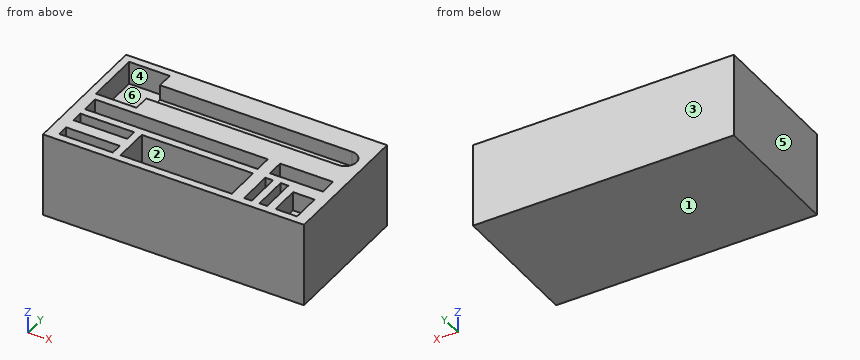
```python
from build123d import *

# Parameters (mm, degrees)
F0_W      = 340
F0_H      = 180
F1_DEPTH  = 110
F2_W      = 53
F2_H      = 72
F4_DEPTH  = 30
F5_DEPTH  = 20
F7_W      = 225
F7_H      = 22
F12_DEPTH = 100
F6_W      = 70
F6_H      = 15
F13_DEPTH = 80
F8_W      = 145
F8_H      = 46
F14_DEPTH = 100
F9_W      = 69
F9_H      = 22
F15_DEPTH = 100
F10_W     = 10
F10_H     = 46
F16_DEPTH = 15
F11_W     = 28
F11_H     = 38
F17_DEPTH = 25


with BuildPart() as f1:
    # F0 (on Top) → F1 (new body)
    with BuildSketch(Plane.XY):
        Rectangle(F0_W, F0_H)
    extrude(amount=-F1_DEPTH)

    # F2 (on face) → F4 (cut)
    with BuildSketch(Plane.XY):
        with Locations((-133.5, 44)):
            Rectangle(F2_W, F2_H)
    extrude(amount=-F4_DEPTH, mode=Mode.SUBTRACT)

    # F3 (on face) → F5 (cut)
    with BuildSketch(Plane.XY):
        with BuildLine():
            Line((143, 59), (-107, 59))
            Line((-107, 59), (-107, 29))
            Line((-107, 29), (143, 29))
            ThreePointArc((143, 29), (158, 44), (143, 59))
        make_face()
    extrude(amount=-F5_DEPTH, mode=Mode.SUBTRACT)

    # F7 (on face) → F12 (cut)
    with BuildSketch(Plane.XY):
        with Locations((-42.5, -13)):
            Rectangle(F7_W, F7_H)
    extrude(amount=-F12_DEPTH, mode=Mode.SUBTRACT)

    # F6 (on face) → F13 (cut)
    with BuildSketch(Plane.XY):
        with Locations((-120, -72.5)):
            Rectangle(F6_W, F6_H)
        with Locations((-120, -41.5)):
            Rectangle(F6_W, F6_H)
    extrude(amount=-F13_DEPTH, mode=Mode.SUBTRACT)

    # F8 (on face) → F14 (cut)
    with BuildSketch(Plane.XY):
        with Locations((-2.5, -57)):
            Rectangle(F8_W, F8_H)
    extrude(amount=-F14_DEPTH, mode=Mode.SUBTRACT)

    # F9 (on face) → F15 (cut)
    with BuildSketch(Plane.XY):
        with Locations((120.5, -13)):
            Rectangle(F9_W, F9_H)
    extrude(amount=-F15_DEPTH, mode=Mode.SUBTRACT)

    # F10 (on face) → F16 (cut)
    with BuildSketch(Plane.XY):
        with Locations((91, -57)):
            Rectangle(F10_W, F10_H)
        with Locations((111, -57)):
            Rectangle(F10_W, F10_H)
    extrude(amount=-F16_DEPTH, mode=Mode.SUBTRACT)

    # F11 (on face) → F17 (cut)
    with BuildSketch(Plane.XY):
        with Locations((141, -61)):
            Rectangle(F11_W, F11_H)
    extrude(amount=-F17_DEPTH, mode=Mode.SUBTRACT)


solid = f1.part
```
Work out the finished part from the listing and answer in its coordinate system (mm). Face numbers are marked on the shaded views. A direction names the side the tool comes from. Coordinates: 2 decimals unless noted, no trailing zeros. Write each loop counter-clockwise with the first axis right and the second up, starting at its lowest first coordinate (ties: lowest second). Pieces come first, ordered by that corner, then holes. Notation, with made-up numbers: (72.5, -10) - (84.5, -10) arc R29 cw to (84.5, 20) - close; hole circle Ø8 at (-30, 42). An arc over 180 degrees is marked (long way). Answer as a JSON object with one key per item and string values.
Q1. Find section D-D (y = -5.5). Write down the section's boundary in (x, z), plus the area to 3 significant figures.
Results list:
{"outline": "(-170, -110) - (170, -110) - (170, 0) - (155, 0) - (155, -100) - (86, -100) - (86, 0) - (70, 0) - (70, -100) - (-155, -100) - (-155, 0) - (-170, 0) - close", "area": "8,000 mm^2"}
Q2. Find section B-B (x = 133). Write down the section's boundary in (y, z).
Results list:
{"outline": "(-90, -110) - (90, -110) - (90, 0) - (59, 0) - (59, -20) - (29, -20) - (29, 0) - (-2, 0) - (-2, -100) - (-24, -100) - (-24, 0) - (-42, 0) - (-42, -25) - (-80, -25) - (-80, 0) - (-90, 0) - close"}
Q3. Which of the six approach directions +Z, -Z, +X, -X, +Y, -Y give full straight-line access (tool end or side, diameter ignored) to the marked faces 5 and 6?
Results list:
{"face 5": "+Z, -Z, -X, +Y, -Y", "face 6": "+Z"}
Q4. Find section A-A (z = -43.5). Write down the section's boundary in (x, y), plus the area to 3 significant figures.
Results list:
{"outline": "(-170, -90) - (170, -90) - (170, 90) - (-170, 90) - close; hole (-155, -80) - (-85, -80) - (-85, -65) - (-155, -65) - close; hole (-155, -49) - (-85, -49) - (-85, -34) - (-155, -34) - close; hole (-155, -24) - (70, -24) - (70, -2) - (-155, -2) - close; hole (-75, -80) - (70, -80) - (70, -34) - (-75, -34) - close; hole (86, -24) - (155, -24) - (155, -2) - (86, -2) - close", "area": "46,000 mm^2"}
Q5. Consider L1, parallel to Y at x = 67.5, z = -25; L2, parallel to Y at x = -93, z = -47; L3, parallel to Y at x = -91.5, z = -5.5. Determine where each line is inside the solid, lowest interval first. Write a range as from..to.
Results list:
{"L1": "y = -90..-80, -34..-24, -2..90", "L2": "y = -90..-80, -65..-49, -34..-24, -2..90", "L3": "y = -90..-80, -65..-49, -34..-24, -2..29, 59..90"}
Q6. For a pull along Y with two mould halves and no side action, classify the marked faces 1, 2, 3 and 4 as pulls with the +Y half, pulls with the -Y half, needs draft (parallel to the pull), parting line crosses it, or undercut.
Results list:
{"face 1": "needs draft", "face 2": "undercut", "face 3": "pulls with the +Y half", "face 4": "undercut"}
Q7. Find section C-C (y = 44). Write down the section's boundary in (x, z), plus the area to 3 significant figures.
Results list:
{"outline": "(-170, -110) - (170, -110) - (170, 0) - (158, 0) - (158, -20) - (-107, -20) - (-107, -30) - (-160, -30) - (-160, 0) - (-170, 0) - close", "area": "30,500 mm^2"}
Q8. Given pin 1 Ø5 at (x, y) = (49.5, 52) entering from +Z; pin 2 Ø11 at (x, y) = (136.5, -15.5) entering from +Z; pin 3 Ø7.5 at (x, y) = (-119, -71.5) entering from +Z, each flat-ended and moving along its own axis, determine where each tip first touches the part or whether it passes through.
Results list:
{"pin 1": "stops at z = -20", "pin 2": "stops at z = -100", "pin 3": "stops at z = -80"}
